```python
from build123d import *

# Parameters (mm, degrees)
BOSS_EXTRUDE1_START = 19.16
SKETCH1_W           = 90
SKETCH1_H           = 100
SKETCH1_R           = 2.5
SKETCH1_R_2         = 3.57
BOSS_EXTRUDE1_DEPTH = 3.18
SKETCH2_W           = 45.72
SKETCH2_H           = 65.511870912
CUT_EXTRUDE1_DEPTH  = 72.134467033
FILLET1_R           = 10


with BuildPart() as part:
    # Sketch1 → Boss-Extrude1 (new body)
    with BuildSketch(Plane.XY.offset(BOSS_EXTRUDE1_START)):
        with Locations((0, -5)):
            Rectangle(SKETCH1_W, SKETCH1_H)
        with Locations((32.3, -12.3)):
            Circle(SKETCH1_R, mode=Mode.SUBTRACT)
        with Locations((32.3, -42.3)):
            Circle(SKETCH1_R, mode=Mode.SUBTRACT)
        with Locations((-32.3, -42.3)):
            Circle(SKETCH1_R_2, mode=Mode.SUBTRACT)
        with Locations((-32.3, -12.3)):
            Circle(SKETCH1_R, mode=Mode.SUBTRACT)
        with Locations((-32.3, 32.3)):
            Circle(SKETCH1_R_2, mode=Mode.SUBTRACT)
        with Locations((32.3, 32.3)):
            Circle(SKETCH1_R, mode=Mode.SUBTRACT)
    extrude(amount=-BOSS_EXTRUDE1_DEPTH)

    # Sketch2 → Cut-Extrude1 (cut, through all)
    with BuildSketch(Plane(origin=(0, 0, 15.98), x_dir=(-1, 0, 0), z_dir=(0, 0, -1))):
        with Locations((0, -22.244064544)):
            Rectangle(SKETCH2_W, SKETCH2_H)
    extrude(amount=-CUT_EXTRUDE1_DEPTH, mode=Mode.SUBTRACT)

    # Fillet1
    fillet1_edges = [part.edges().sort_by_distance(p)[0] for p in [
        (22.86, 10.511870912, 17.57),
        (-22.86, 10.511870912, 17.57),
        (-45, 45, 17.57),
        (45, 45, 17.57),
        (45, -55, 17.57),
        (-45, -55, 17.57),
    ]]
    fillet(fillet1_edges, radius=FILLET1_R)


solid = part.part
```
The listing builds one solid part. Answer for the finished solid, in the listing's coordinates (mm). A direction names the side the tool comes from. Give positions to 0.01 mm unless a question says otherwise; leave off trailing zeros. Order: outer loops, then holes, each group sorted by start corner. A loop starts at its lowest first (then second) coordinate and runs counter-clockwise, first axis right, second up.
Item 1: Find the intervals of material crossed by probe 1 along Y at (x, z) = (32.3, 18.5); probe 2 along Y at (x, z) = (-32.3, 17.6); probe 3 along X at (y, z) = (30.5, 16.7), in increasing order.
From the geometry:
probe 1: y = -55 to -44.8, -39.8 to -14.8, -9.8 to 29.8, 34.8 to 45
probe 2: y = -55 to -45.87, -38.73 to -14.8, -9.8 to 28.73, 35.87 to 45
probe 3: x = -45 to -35.38, -29.22 to 30.57, 34.03 to 45
Item 2: Given pin 1 Ø1 at (x, z) = (5, 18.5) entering from -Y; pin 2 Ø5.5 at (x, y) = (-32.3, 32.3) entering from -Z, each flat-ended and moving along its own axis, determine where each tip first touches the part or whether it passes through.
From the geometry:
pin 1: stops at y = 10.51
pin 2: passes through
Item 3: The part is cut by section B-B, the plane y = -12.3. Give the vertices of the cut face in (x, z), and give its area (3 significant figures).
From the geometry:
outline: (-45, 15.98) - (-34.8, 15.98) - (-34.8, 19.16) - (-45, 19.16) - close; (-29.8, 15.98) - (-22.86, 15.98) - (-22.86, 19.16) - (-29.8, 19.16) - close; (22.86, 15.98) - (29.8, 15.98) - (29.8, 19.16) - (22.86, 19.16) - close; (34.8, 15.98) - (45, 15.98) - (45, 19.16) - (34.8, 19.16) - close
area: 109 mm2
Item 4: The part is cut by section D-D, the plane y = 32.3. Give the vertices of the cut face in (x, z).
From the geometry:
outline: (-45, 15.98) - (-35.87, 15.98) - (-35.87, 19.16) - (-45, 19.16) - close; (-28.73, 15.98) - (29.8, 15.98) - (29.8, 19.16) - (-28.73, 19.16) - close; (34.8, 15.98) - (45, 15.98) - (45, 19.16) - (34.8, 19.16) - close
Item 5: The part is cut by section A-A, the plane x = 32.3. Give the vertices of the cut face in (y, z).
From the geometry:
outline: (-55, 15.98) - (-44.8, 15.98) - (-44.8, 19.16) - (-55, 19.16) - close; (-39.8, 15.98) - (-14.8, 15.98) - (-14.8, 19.16) - (-39.8, 19.16) - close; (-9.8, 15.98) - (29.8, 15.98) - (29.8, 19.16) - (-9.8, 19.16) - close; (34.8, 15.98) - (45, 15.98) - (45, 19.16) - (34.8, 19.16) - close
Item 6: The part is cut by section C-C, the plane z = 18.4. Give the vertices of the cut face in (x, y), and give its area (3 significant figures).
From the geometry:
outline: (-45, -45) arc R10 ccw to (-35, -55) - (-22.86, -55) - (-22.86, 0.51) arc R10 cw to (-12.86, 10.51) - (12.86, 10.51) arc R10 cw to (22.86, 0.51) - (22.86, -55) - (35, -55) arc R10 ccw to (45, -45) - (45, 35) arc R10 ccw to (35, 45) - (-35, 45) arc R10 ccw to (-45, 35) - close; hole circle Ø7.14 at (-32.3, -42.3); hole circle Ø7.14 at (-32.3, 32.3); hole circle Ø5 at (-32.3, -12.3); hole circle Ø5 at (32.3, -42.3); hole circle Ø5 at (32.3, -12.3); hole circle Ø5 at (32.3, 32.3)
area: 5,800 mm2
Item 7: For a pull along X with two mould halves and no side action, classify faces 1 (the face through (41.99, 42.15, 17.55)), 2 (the face through (0, 10.512, 18)), 3 (the face through (0, 45, 18)), 4 (the face through (-42.15, -51.99, 17.55)) as pulls with the +X half, pulls with the -X half, needs draft (parallel to the pull), parting line crosses it, or undercut.
From the geometry:
face 1: pulls with the +X half
face 2: undercut
face 3: needs draft
face 4: pulls with the -X half
Item 8: Which of the six approach directions +Z, -Z, +X, -X, +Y, -Y give full straight-line access (tool end or side, diameter ignored) to faces 5 (the face through (-20.008, 7.505, 17.592)), 6 (the face through (34.685, -11.549, 17.592))?
From the geometry:
face 5: +Z, -Z, -Y
face 6: +Z, -Z
